from build123d import *

# Parameters (mm, degrees)
SKETCH1_W           = 60
SKETCH1_H           = 15
BOSS_EXTRUDE1_DEPTH = 2
SKETCH2_R           = 4
CUT_EXTRUDE1_DEPTH  = 2
FILLET2_R           = 5


with BuildPart() as part:
    # Sketch1 → Boss-Extrude1 (new body)
    with BuildSketch(Plane(origin=(0, 0, 0), x_dir=(1, 0, 0), z_dir=(0, 1, 0))):
        with Locations((30, 9.203056769)):
            Rectangle(SKETCH1_W, SKETCH1_H)
    extrude(amount=BOSS_EXTRUDE1_DEPTH)

    # Sketch2 → Cut-Extrude1 (cut)
    with BuildSketch(Plane(origin=(0, 2, 0), x_dir=(1, 0, 0), z_dir=(0, 1, 0))):
        with Locations(Location((7, 9.203056769, 0), (0, 0, 270))):
            Circle(SKETCH2_R)
        with Locations(Location((53, 9.203056769, 0), (0, 0, 270))):
            Circle(SKETCH2_R)
    extrude(amount=-CUT_EXTRUDE1_DEPTH, mode=Mode.SUBTRACT)

    # Fillet2
    fillet2_edges = [part.edges().sort_by_distance(p)[0] for p in [
        (0, 1, -16.703056769),
        (60, 1, -16.703056769),
        (60, 1, -1.703056769),
        (0, 1, -1.703056769),
    ]]
    fillet(fillet2_edges, radius=FILLET2_R)


solid = part.part
Part model, mm, in its own coordinate system. Give positions to 0.01 mm unless a question says otherwise; leave off trailing zeros. Loops run counter-clockwise (first coordinate to the right, second up) from the corner with the lowest first, then second, coordinate; pieces in that order, holes last. Notation, with made-up numbers: M 30.25,5.5 L 66.25,5.5 A23 ccw 66.25,26.5 Z; hole C 34.25,-30 d1. An arc over 180 degrees is marked long. Put each result on its own line as item: value. Start each with the question number.
1) Flat gauge pin, fed straight in: pin 1 (1 mm diameter, centred on y = 1.5, z = -12.5, fed in from -X). Where does the tip first touch, or does it go through?
2) Probe probe 1 along X at (y, z) = (1.9, -9.5); probe 2 along X at (y, z) = (1.7, -11.5); probe 3 along Z at (x, y) = (10, 0.95). List the from-to ranges inside material, lowest first.
3) Saw through at B-B (y = 0.95). List the corners of the cut face in (x, z), then the cut area to 3 significant figures.
4) Saw through at D-D (z = -3.5). List the corners of the cut face in (x, y), then the cut area to 3 significant figures.
5) Saw through at C-C (z = -8.5). List the corners of the cut face in (x, y).
6) Pull direction Z, two halves, no side cores. Call faces 1 (the cylindrical face through (58.496, 1.014, -15.277)), 2 (the flat face through (60, 1, -9)), 3 (the cylindrical face through (7.2, 1, -13.2)): +Z half, -Z half, draft (parallel to the pull), parting line (faces both ways), or undercut.
7) Saw through at A-A (x = 7). List the corners of the cut face in (y, z).
Numbers:
1. pin 1: x = 0.01
2. probe 1: 0 to 3.01, 10.99 to 49.01, 56.99 to 60
2. probe 2: 0 to 3.73, 10.27 to 49.73, 56.27 to 60
2. probe 3: -16.7 to -11.85, -6.56 to -1.7
3. outline: M 0,-11.7 A5 ccw 5,-16.7 L 55,-16.7 A5 ccw 60,-11.7 L 60,-6.7 A5 ccw 55,-1.7 L 5,-1.7 A5 ccw 0,-6.7 Z; hole C 7,-9.2 d8; hole C 53,-9.2 d8
3. area: 778 mm^2
4. outline: M 1.16,0 L 58.84,0 L 58.84,2 L 1.16,2 Z
4. area: 115 mm^2
5. outline: M 0,0 L 3.06,0 L 3.06,2 L 0,2 Z; M 10.94,0 L 49.06,0 L 49.06,2 L 10.94,2 Z; M 56.94,0 L 60,0 L 60,2 L 56.94,2 Z
6. face 1: -Z half
6. face 2: draft
6. face 3: undercut
7. outline: M 0,-16.7 L 2,-16.7 L 2,-13.2 L 0,-13.2 Z; M 0,-5.2 L 2,-5.2 L 2,-1.7 L 0,-1.7 Z
